Job drawing, mm, ordinate dimensions from the low corner. One solid piece. Give positions to 0.01 mm unless a question says otherwise; leave off trailing zeros. Write each loop counter-clockwise with the first axis right and the second up, starting at its lowest first coordinate (ties: lowest second). Pieces come first, ordered by that corner, then holes. Notation, with made-up numbers: M 17.5,23.5 L 53.5,23.5 A29 ccw 53.5,55.5 Z; hole C 82.5,-17 d5. An arc over 180 degrees is marked long. Answer as CSV lines item,"result". Start each with the question number.
1) Slice it at B-B, the plane y = 29. Give the cut face in (x, z), plus the area to 3 significant figures.
2) Wall check: line 1 along Y through (x, z) = (46, 26); line 2 along Z through (x, y) = (44, 17.5); line 3 along Y through (x, z) = (25, 3.3). Give the ranges that are in metal, low to high. Write a range as from..to.
3) Mould opens along Y. For the marked faces 1 and 2 say: pulls with the +Y half, pulls with the -Y half, needs draft (parallel to the pull), parting line crosses it, or undercut.
4) Slice it at C-C, the plane x = 104. Give the cut face in (y, z), plus the area to 3 significant figures.
5) Pin check, flat tips, straight feed: pin 1 Ø12 at (y, z) = (36.5, 17) entering from +X; pin 2 Ø1 at (x, y) = (106, 27) entering from +Z; pin 3 Ø4 at (x, z) = (19.5, 7) entering from -Y; pin 4 Ø2 at (x, z) = (56, 22.5) entering from +Y. Stop position of each tip, or through.
6) Slice it at A-A, the plane z = 25. Give the cut face in (x, y), plus the area to 3 significant figures.
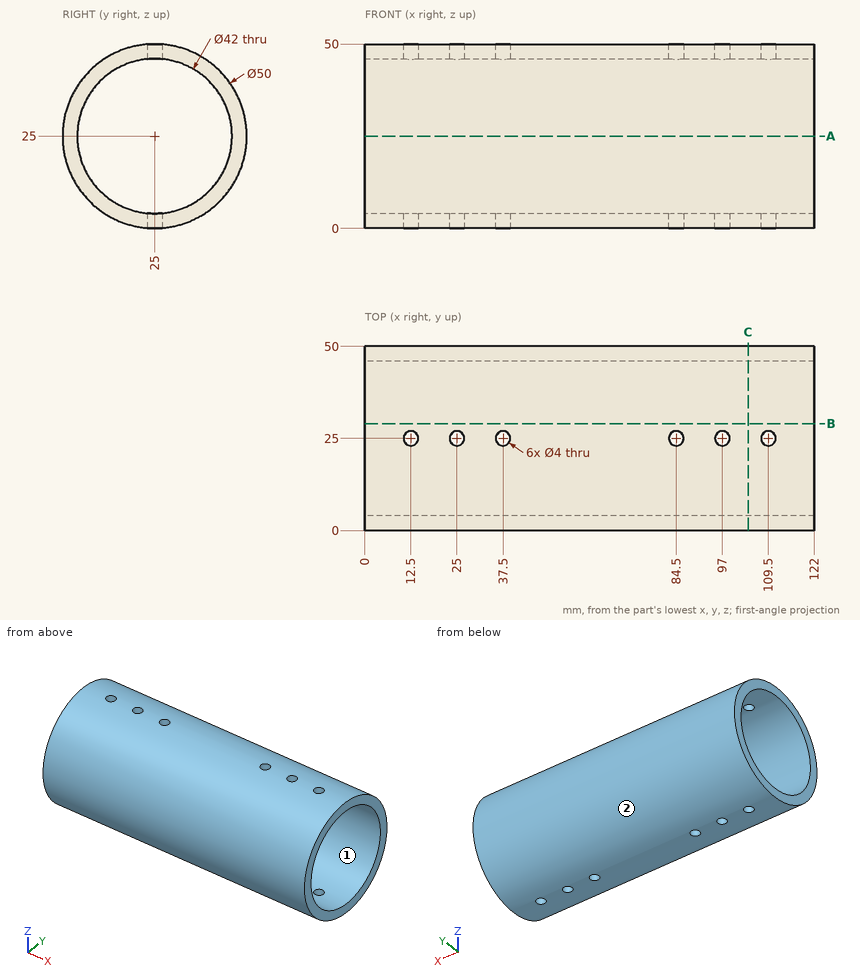
Found:
1,outline,"M 0,0.32 L 122,0.32 L 122,4.38 L 0,4.38 Z; M 0,45.62 L 122,45.62 L 122,49.68 L 0,49.68 Z"
1,area,"991 mm²"
2,line 1,"0.02..4.02, 45.98..49.98"
2,line 2,"1.15..5.38, 44.62..48.85"
2,line 3,"12.59..23, 27..37.41"
3,face 1,"undercut"
3,face 2,"parting line crosses it"
4,outline,"C 25,25 d50; hole C 25,25 d42"
4,area,"578 mm²"
5,pin 1,"through"
5,pin 2,"z = 49.95"
5,pin 3,"y = 5.79"
5,pin 4,"y = 49.95"
6,outline,"M 0,0 L 122,0 L 122,4 L 0,4 Z; M 0,46 L 122,46 L 122,50 L 0,50 Z"
6,area,"976 mm²"
